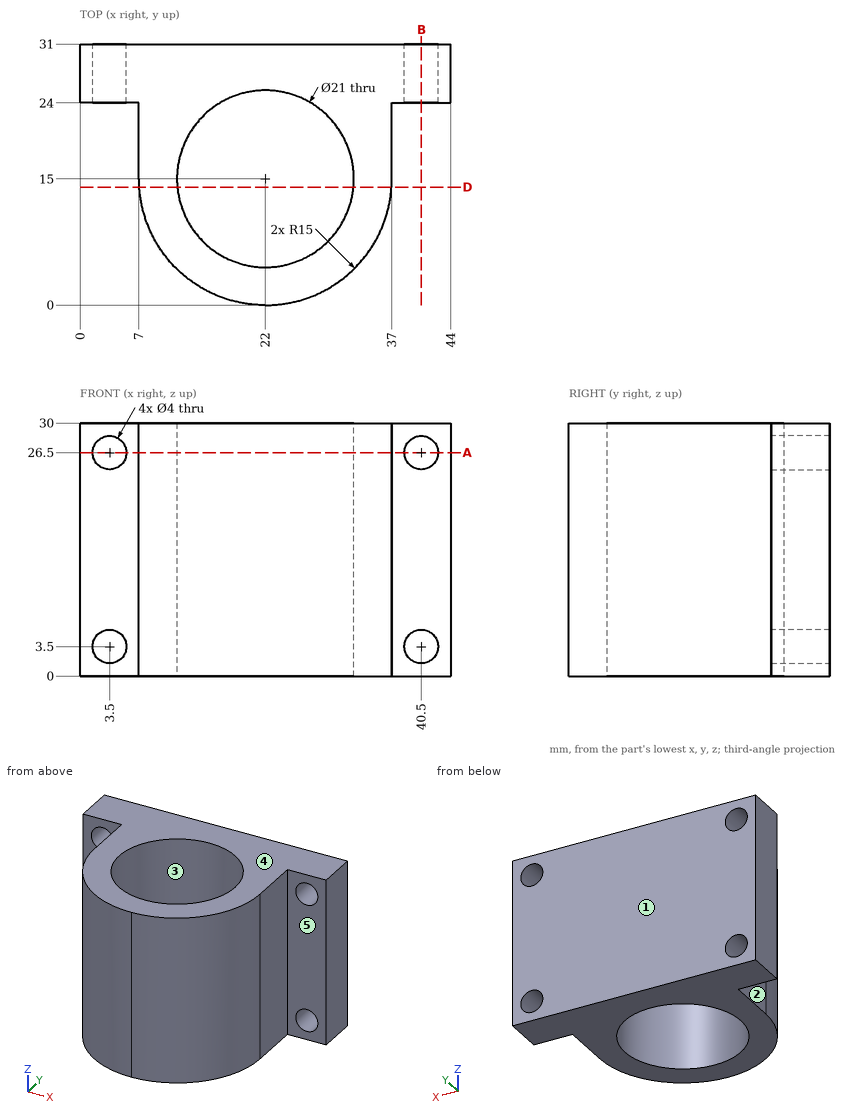
Answer from the drawing. Dimensions are ordinates in mm from the lowest x, y and z of the part. A direction names the side the tool comes from. Give positions to 0.01 mm unless a question says otherwise; leave off trailing zeros. Loops run counter-clockwise (first coordinate to the right, second up) from the corner with the lowest first, then second, coordinate; pieces in that order, holes last.
Item 1: A cutting plane is placed at B-B (x = 40.5). Give the vertices of the cut face in (y, z).
Derived:
outline: (24, 0) - (31, 0) - (31, 1.5) - (24, 1.5) - close; (24, 5.5) - (31, 5.5) - (31, 24.5) - (24, 24.5) - close; (24, 28.5) - (31, 28.5) - (31, 30) - (24, 30) - close
Item 2: A cutting plane is placed at D-D (y = 14). Give the vertices of the cut face in (x, z).
Derived:
outline: (7.03, 0) - (11.55, 0) - (11.55, 30) - (7.03, 30) - close; (32.45, 0) - (36.97, 0) - (36.97, 30) - (32.45, 30) - close
Item 3: Find the intervals of material crossed by line 1 along X through (y, z) = (28.75, 26.5); line 2 along Z through (x, y) = (40, 28); line 3 along Y through (x, z) = (39, 16), in increasing order.
Derived:
line 1: x = 0 to 1.5, 5.5 to 38.5, 42.5 to 44
line 2: z = 0 to 1.56, 5.44 to 24.56, 28.44 to 30
line 3: y = 24 to 31
Item 4: A cutting plane is placed at A-A (z = 26.5). Give the number of separate pieces and of enclosed holes in the cut face, then the cut area to 3 significant figures.
Derived:
separate pieces: 3
enclosed holes: 1
area: 529 mm2
Item 5: Each of these flat-tipped pins is pushed along its axis until it touches: pin 1 Ø7.5 at (x, z) = (39, 10.5) entering from -Y; pin 2 Ø3 at (x, z) = (40.5, 3.5) entering from +Y; pin 3 Ø1.5 at (y, z) = (12, 11) entering from -X; pin 4 Ø12 at (x, z) = (33.5, 8.5) entering from -Y. Where does it stop, or does it pass through?
Derived:
pin 1: stops at y = 7.97
pin 2: passes through
pin 3: stops at x = 7.17
pin 4: stops at y = 1.04
Item 6: Determine the mould class of the marked faces 1, 2 and 3 for opening direction X: +X half, -X half, draft (parallel to the pull), parting line (faces both ways), or undercut.
Derived:
face 1: draft
face 2: -X half
face 3: undercut
Item 7: A tool of negligible diameter and unlimited length cuts with its end or side. For the marked faces 4 and 5, from which of +Z, -Z, +X, -X, +Y, -Y can it reach the whole face along a straight path? Write none if from no direction.
Derived:
face 4: +Z, +X, -X, +Y, -Y
face 5: +Z, -Z, +X, -Y
